```python
from build123d import *

# Parameters (mm, degrees)
F0_W     = 63.5
F0_H     = 63.5
F1_DEPTH = 25.4
F2_R     = 12.7


with BuildPart() as f1:
    # F0 (on Front) → F1 (new body)
    with BuildSketch(Plane.XZ):
        with Locations((31.75, 31.75)):
            Rectangle(F0_W, F0_H)
        with BuildLine():
            ThreePointArc((19.05, 12.7), (13.648367, 15.711607), (13.370387, 21.889806))
            Line((13.370387, 21.889806), (26.070387, 47.289806))
            ThreePointArc((26.070387, 47.289806), (31.75, 50.8), (37.429613, 47.289806))
            Line((37.429613, 47.289806), (50.129613, 21.889806))
            ThreePointArc((50.129613, 21.889806), (49.851633, 15.711607), (44.45, 12.7))
            Line((44.45, 12.7), (19.05, 12.7))
        make_face(mode=Mode.SUBTRACT)
    extrude(amount=F1_DEPTH)

    # F2
    f2_edges = [f1.edges().sort_by_distance(p)[0] for p in [
        (63.5, -12.7, 63.5),
        (0, -12.7, 63.5),
        (0, -12.7, 0),
        (63.5, -12.7, 0),
    ]]
    fillet(f2_edges, radius=F2_R)


solid = f1.part
```
Check sheet for the modelled part. Datum: model origin and axes. Units: mm. A direction names the side the tool comes from. Round coordinates to 2 decimals unless told otherwise and drop trailing zeros. Write each loop counter-clockwise with the first axis right and the second up, starting at its lowest first coordinate (ties: lowest second). Pieces come first, ordered by that corner, then holes. Notation, with made-up numbers: M 50,2.5 L 95,2.5 A17 ccw 95,15.5 Z; hole C 19,35.25 d8. An arc over 180 degrees is marked long. Write item = value, one per line. Start each with the question number.
1. Release check for a two-part mould opening along X. For faces 3 (the flat face through (45.4, -25.4, 32.2)), 4 (the cylindrical face through (31.7, -12.5, 50.8)), 5 (the cylindrical face through (3.62, -12.88, 59.68)), 6 (the cylindrical face through (13.696, -12.522, 15.635)) record: pulls with the +X half, pulls with the -X half, needs draft (parallel to the pull), parting line crosses it, or undercut.
2. Section check A-A, the plane y = -10. Record the cut outline in (x, z), then the cut area to 3 significant figures.
3. Scan lines: line 1 (Z direction, x = 21, y = -11); line 2 (Z direction, x = 25, y = -19.25); line 3 (X direction, y = -13.5, z = 30.5). Record each from-to range of solid material in increasing order. Write a range as [from, to].
4. Section check D-D, the plane z = 5. Record the cut outline in (x, y), then the cut area to 3 significant figures.
5. Section check C-C, the plane x = 39. Record the cut outline in (y, z).
6. Tool access check on faces 1 (the cylindrical face through (49.9, -12.52, 15.79)), 2 (the cylindrical face through (3.62, -12.88, 3.82)). Record the directions out of +Z, -Z, +X, -X, +Y, -Y that give a thin tool (end or side, any length) a straight path to the whole face; none if there is none.
7. Section check B-B, the plane z = 26. Record the cut outline in (x, y), then the cut area to 3 significant figures.
Results found:
q1.face_3 = needs draft
q1.face_4 = undercut
q1.face_5 = pulls with the -X half
q1.face_6 = undercut
q2.outline = M 0,12.7 A12.7 ccw 12.7,0 L 50.8,0 A12.7 ccw 63.5,12.7 L 63.5,50.8 A12.7 ccw 50.8,63.5 L 12.7,63.5 A12.7 ccw 0,50.8 Z; hole M 13.37,21.89 A6.35 ccw 19.05,12.7 L 44.45,12.7 A6.35 ccw 50.13,21.89 L 37.43,47.29 A6.35 ccw 26.07,47.29 Z
q2.area = 2,920 mm^2
q3.line_1 = [0, 12.7], [37.15, 63.5]
q3.line_2 = [0, 12.7], [45.15, 63.5]
q3.line_3 = [0, 17.68], [45.82, 63.5]
q4.outline = M 2.6,-25.4 L 60.9,-25.4 L 60.9,0 L 2.6,0 Z
q4.area = 1,480 mm^2
q5.outline = M -25.4,0 L 0,0 L 0,12.7 L -25.4,12.7 Z; M -25.4,44.15 L 0,44.15 L 0,63.5 L -25.4,63.5 Z
q6.face_1 = +Y, -Y
q6.face_2 = -Z, -X, +Y, -Y
q7.outline = M 0,-25.4 L 15.43,-25.4 L 15.43,0 L 0,0 Z; M 48.07,-25.4 L 63.5,-25.4 L 63.5,0 L 48.07,0 Z
q7.area = 784 mm^2
